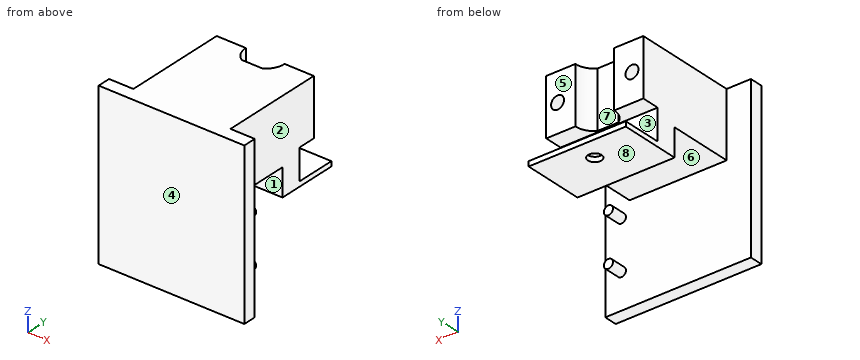
from build123d import *

# Parameters (mm, degrees)
SKETCH_2_W          = 50
SKETCH_2_H          = 4
EXTRUDE_2_DEPTH     = 22.5
SKETCH_15_R         = 1.4
EXTRUDE_8_DEPTH     = 5
SKETCH_3_W          = 30
SKETCH_3_H          = 20
EXTRUDE_4_DEPTH     = 20
EXTRUDE_9_DEPTH     = 17.5
EXTRUDE_10_DEPTH    = 15
CUT_EXTRUDE_1_REACH = 58.089
SKETCH_19_R         = 2.1
SKETCH_20_R         = 2
CUT_EXTRUDE_2_DEPTH = 10


with BuildPart() as part:
    # 草圖2 → 填料-伸長2 (new, symmetric)
    with BuildSketch(Plane(origin=(0, 0, 0), x_dir=(0, 0, -1), z_dir=(1, 0, 0))):
        with Locations((25, 2)):
            Rectangle(SKETCH_2_W, SKETCH_2_H)
    extrude(amount=EXTRUDE_2_DEPTH, both=True)

    # 草圖15 → 填料-伸長8 (add)
    with BuildSketch(Plane(origin=(0, 4, 0), x_dir=(1, 0, 0), z_dir=(0, 1, 0))):
        with Locations(Location((17.5, 39.2, 0), (0, 0, 90))):
            Circle(SKETCH_15_R)
        with Locations(Location((17.5, 24.2, 0), (0, 0, 90))):
            Circle(SKETCH_15_R)
    extrude(amount=EXTRUDE_8_DEPTH)

    # 草圖3 → 填料-伸長4 (add)
    with BuildSketch(Plane(origin=(0, 4, 0), x_dir=(1, 0, 0), z_dir=(0, 1, 0))):
        with Locations((0, 10)):
            Rectangle(SKETCH_3_W, SKETCH_3_H)
    extrude(amount=EXTRUDE_4_DEPTH)

    # 草圖16 → 填料-伸長9 (add)
    with BuildSketch(Plane(origin=(0, 0, 0), x_dir=(-1, 0, 0), z_dir=(0, 0, -1))):
        with BuildLine():
            Line((-15, 24), (-15, 36.000002525))
            Line((-15, 36.000002525), (-6, 36.000002525))
            ThreePointArc((-6, 36.000002525), (-5.267141914, 33.146824473), (-3.25, 31.000002525))
            Line((-3.25, 31.000002525), (3.25, 31.000002525))
            ThreePointArc((3.25, 31.000002525), (5.267141914, 33.146824473), (6, 36.000002525))
            Line((6, 36.000002525), (15, 36.000002525))
            Line((15, 36.000002525), (15, 24))
            Line((15, 24), (-15, 24))
        make_face()
    extrude(amount=EXTRUDE_9_DEPTH)

    # 草圖18 → 填料-伸長10 (add, symmetric)
    with BuildSketch(Plane(origin=(0, 0, 0), x_dir=(0, 0, -1), z_dir=(1, 0, 0))):
        Polygon((17.5, 24), (28.5, 24), (28.5, 42.748788628), (27, 42.748788628), (27, 30.5), (17.5, 30.5), align=None)
    extrude(amount=EXTRUDE_10_DEPTH, both=True)

    # 草圖19 → 除料-伸長1 (cut, up to next)
    with BuildSketch(Plane(origin=(0, 0, -28.5), x_dir=(-1, 0, 0), z_dir=(0, 0, -1)), mode=Mode.PRIVATE) as cut_extrude_1_sk1:
        with Locations((0, 36.000002505)):
            Circle(SKETCH_19_R)
    cut_extrude_1_tool1 = extrude(cut_extrude_1_sk1.sketch, amount=-CUT_EXTRUDE_1_REACH, mode=Mode.PRIVATE) & part.part
    add(cut_extrude_1_tool1.solids().sort_by_distance((0, 36.000003, -28.5))[0], mode=Mode.SUBTRACT)

    # 草圖20 → 除料-伸長2 (cut)
    with BuildSketch(Plane(origin=(0, 36.000002525, 0), x_dir=(1, 0, 0), z_dir=(0, 1, 0))):
        with Locations(Location((-11.5, 8.75, 0), (0, 0, 180))):
            Circle(SKETCH_20_R)
        with Locations(Location((11.5, 8.75, 0), (0, 0, 180))):
            Circle(SKETCH_20_R)
    extrude(amount=-CUT_EXTRUDE_2_DEPTH, mode=Mode.SUBTRACT)


solid = part.part
Part model, mm, in its own coordinate system. Face numbers are marked on the shaded views. A direction names the side the tool comes from. Give positions to 0.01 mm unless a question says otherwise; leave off trailing zeros. Loops run counter-clockwise (first coordinate to the right, second up) from the corner with the lowest first, then second, coordinate; pieces in that order, holes last.
(1) Band-saw the part on A-A (y = 35). Write the cut outline in (x, z), and give its area (3 significant figures).
Return value:
outline: (-15, -28.5) - (-1.85, -28.5) - (-1.85, -27) - (-15, -27) - close; (-15, -17.5) - (-5.91, -17.5) - (-5.91, 0) - (-15, 0) - close; (1.85, -28.5) - (15, -28.5) - (15, -27) - (1.85, -27) - close; (5.91, -17.5) - (15, -17.5) - (15, 0) - (5.91, 0) - close; hole circle Ø4 at (-11.5, -8.75); hole circle Ø4 at (11.5, -8.75)
area: 332 mm2
(2) Pull direction Y, two halves, no side cores. Call the marked faces 1, 2, 3 and 4: pulls with the +Y half, pulls with the -Y half, needs draft (parallel to the pull), parting line crosses it, or undercut.
Return value:
face 1: undercut
face 2: needs draft
face 3: pulls with the +Y half
face 4: pulls with the -Y half
(3) Drill centre lines: line 1 along Y through (x, z) = (0, -28); line 2 along Z through (x, y) = (-11.5, 35.5); line 3 along X through (y, z) = (29, -8). Where is each one in solid material? Low to high.
Return value:
line 1: y = 0 to 4, 24 to 33.9, 38.1 to 42.75
line 2: z = -28.5 to -27, -17.5 to -10.75, -6.75 to 0
line 3: x = -15 to -13.35, -9.65 to 9.65, 13.35 to 15
(4) Band-saw the part on B-B (z = -24.2). Write the cut outline in (x, y), and give its area (3 significant figures).
Return value:
outline: (-22.5, 0) - (22.5, 0) - (22.5, 4) - (18.9, 4) - (18.9, 9) - (16.1, 9) - (16.1, 4) - (-22.5, 4) - close; (-15, 24) - (15, 24) - (15, 30.5) - (-15, 30.5) - close
area: 389 mm2
(5) Band-saw the part on C-C (x = 11.5). Write the cut outline in (y, z).
Return value:
outline: (0, -50) - (4, -50) - (4, -20) - (24, -20) - (24, -28.5) - (42.75, -28.5) - (42.75, -27) - (30.5, -27) - (30.5, -17.5) - (36, -17.5) - (36, -10.75) - (26, -10.75) - (26, -6.75) - (36, -6.75) - (36, 0) - (0, 0) - close
(6) 3-axis set-ups, long thin cutter, end or side, ignore diameter. For the marked faces 5, 6, 7 and 8: which of +Z, -Z, +X, -X, +Y, -Y reach the whole face in a straight line?
Return value:
face 5: +Z, +X, -X, +Y
face 6: -Z, +X, -X
face 7: +Z, +Y
face 8: -Z, +X, -X, +Y
(7) Pin check, flat tips, straight feed: pin 1 (5 mm diameter, centred on x = 1, z = -26, fed in from -Y); pin 2 (8 mm diameter, centred on x = -6, y = 17, fed in from -Z); pin 3 (3 mm diameter, centred on x = 18, z = -24.5, fed in from +Y); pin 4 (3.5 mm diameter, centred on x = 11.5, z = -8.75, fed in from +Y). Stop position of each tip, or through.
Return value:
pin 1: stops at y = 0
pin 2: stops at z = -20
pin 3: stops at y = 9
pin 4: stops at y = 26
(8) Band-saw the part on D-D (y = 27.5). Write the cut outline in (x, z).
Return value:
outline: (-15, -28.5) - (15, -28.5) - (15, 0) - (-15, 0) - close; hole circle Ø4 at (-11.5, -8.75); hole circle Ø4 at (11.5, -8.75)
